Here's how the part is built. I have some questions about the finished solid (model axes, mm). Round coordinates to 2 decimals unless told otherwise and drop trailing zeros. Loops run counter-clockwise (first coordinate to the right, second up) from the corner with the lowest first, then second, coordinate; pieces in that order, holes last. Notation, with made-up numbers: M 72.25,-4.75 L 88.25,-4.75 A5 ccw 88.25,3.25 Z; hole C 48.5,-32 d3. An arc over 180 degrees is marked long. Use a Markdown table: item, result.
from build123d import *

# Parameters (mm, degrees)
F0_W     = 75.351886
F0_H     = 90.236254
F0_W_2   = 75.087629
F2_DEPTH = 25.4
F1_R     = 12.629289
F3_ANGLE = -180


with BuildPart() as f2:
    # F0 (on Top) → F2 (new body)
    with BuildSketch(Plane.XY):
        with Locations((37.675943, 0)):
            Rectangle(F0_W, F0_H)
        with Locations((-37.543814, 0)):
            Rectangle(F0_W_2, F0_H)
    extrude(amount=-F2_DEPTH)

    # F1 (on face) → F3 (revolve)
    with BuildSketch(Plane.XY):
        with Locations((60.014084, 0)):
            Circle(F1_R)
    revolve(axis=Axis((0, 0.875765, 0), (0, 1, 0)), revolution_arc=F3_ANGLE)


solid = f2.part
1. I need wall thicknesses on probe 1 along Z at (x, y) = (-31, 20); probe 2 along X at (y, z) = (0, 15); probe 3 along X at (y, z) = (7, 28). Which ranges of each line are inside material? Lowest first, please. Write a range as from..to.
Answer sheet:
| item | result |
|---|---|
| probe 1 | -25.4..0 |
| probe 2 | -71.08..-44.95, 44.95..71.08 |
| probe 3 | -64.73..-40.82, 40.82..64.73 |
2. Imagine slicing it at B-B, the plane y = -33. Write out the boundary of the cut face in (x, z), then the cut area to 3 significant figures.
Answer sheet:
| item | result |
|---|---|
| outline | M -75.09,-25.4 L 75.35,-25.4 L 75.35,0 L -75.09,0 Z |
| area | 3,820 mm2 |
3. For pin 1 Ø4 at (y, z) = (1.5, 53) entering from -X; pin 2 Ø8 at (x, y) = (-29.5, -19.5) entering from +Z, each with a flat end and sliding along its axis, tell me the tip position at first contact or that it passes through.
Answer sheet:
| item | result |
|---|---|
| pin 1 | x = -51.63 |
| pin 2 | z = 0 |
4. Imagine slicing it at A-A, the plane y = -4. Write out the boundary of the cut face in (x, z).
Answer sheet:
| item | result |
|---|---|
| outline | M -75.09,-25.4 L 75.35,-25.4 L 75.35,0 L 71.99,0 A71.99 ccw -71.99,0 L -75.09,0 Z; hole M -48.03,0 L 48.03,0 A48.03 ccw Z |
5. We'd pull the mould along X, two halves only. Please class faces 1 (the face through (-75.088, -1, -13)), 2 (the face through (1, 45.118, -13)), 3 (the face through (-1, 1, 0)): +X half, -X half, draft (parallel to the pull), parting line (faces both ways), or undercut.
Answer sheet:
| item | result |
|---|---|
| face 1 | -X half |
| face 2 | draft |
| face 3 | undercut |
